Autodesk Inventor part; units mm, degrees
ref_plane "YZ Plane" through (0, 0, 0) normal (1, 0, 0) x (0, 1, 0)
ref_plane "XZ Plane" through (0, 0, 0) normal (0, 1, 0) x (-1, 0, 0)
ref_plane "XY Plane" through (0, 0, 0) normal (0, 0, 1) x (1, 0, 0)
sketch "Sketch1" plane through (0, 0, 0) normal (0, 1, 0) x (-1, 0, 0)
  line L0 (0, 0) -> (1219.2, 0)
  line L1 (1219.2, 0) -> (1219.2, -1219.2)
  line L2 (1219.2, -1219.2) -> (0, -1219.2)
  line L3 (0, -1219.2) -> (0, 0)
  dimension "d0" = 1219.2
  dimension "d1" = 1219.2
extrude "Extrusion1" add sketch "Sketch1" along normal blind 25.4
sketch "Sketch2" plane through (0, 25.4, 0) normal (0, 1, 0) x (1, 0, 0)
  line L0 (-790.7708, 108.1811) -> (-790.7708, 1049.4054)
  line L1 (-790.7708, 1049.4054) -> (-104.9708, 1049.4054)
  line L2 (-104.9708, 1049.4054) -> (-104.9708, 656.4029)
  line L3 (-104.9708, 656.4029) -> (-468.5932, 656.4029)
  line L4 (-468.5932, 656.4029) -> (-468.5932, 108.1811)
  line L5 (-468.5932, 108.1811) -> (-790.7708, 108.1811)
  point P0 (0, 0)
  dimension "d10" = 685.8
extrude "Extrusion2" add sketch "Sketch2" along normal blind 304.8
sketch "Sketch3" plane through (-104.9708, 25.4, -656.4029) normal (1, 0, 0) x (0, 0, -1)
  line L0 (-33.1569, 274.7838) -> (196.5012, 492.1801)
  line L1 (196.5012, 492.1801) -> (437.777, 274.7838)
  line L2 (437.777, 274.7838) -> (-33.1569, 274.7838)
  line L3 (0, 304.8) -> (393.0024, 304.8)
  point P0 (-656.4029, -25.4)
extrude "Extrusion3" add sketch "Sketch3" along normal blind 25.4
extrude "Extrusion4" add sketch "Sketch3" against normal blind 711.2
sketch "Sketch4" plane through (-790.7708, 25.4, -108.1811) normal (0, 0, 1) x (1, 0, 0)
  line L0 (-63.4257, 274.7838) -> (161.0888, 492.1801)
  line L1 (161.0888, 492.1801) -> (386.3126, 274.7838)
  line L2 (322.1776, 274.7838) -> (711.2, 274.7838)
  line L3 (-63.4257, 274.7838) -> (386.3126, 274.7838)
  line L4 (0, 304.8) -> (322.1776, 304.8)
  line L5 (711.2, 492.1801) -> (-25.4, 492.1801)
  point P0 (790.7708, -25.4)
extrude "Extrusion5" add sketch "Sketch4" against normal blind 744.22
extrude "Extrusion6" add sketch "Sketch4" along normal blind 25.4
sketch "Sketch5" plane through (0, 0, 0) normal (0, -1, 0) x (1, 0, 0)
  line L0 (-560.0074, -996.6268) -> (-666.9511, -996.6268)
  line L1 (-666.9511, -996.6268) -> (-666.9511, -948.1994)
  line L2 (-666.9511, -948.1994) -> (-560.0074, -948.1994)
  line L3 (-560.0074, -948.1994) -> (-560.0074, -996.6268)
  point P0 (0, 0)
extrude "Extrusion7" add sketch "Sketch5" against normal blind 508
equation "\"d1\" = d0"
properties part number "house_1" material "Wood (Oak)"
Design review of the part built by this model. Coordinates are the model's own, in mm. A direction names the side the tool comes from. Round coordinates to 2 decimals unless told otherwise and drop trailing zeros. Write each loop counter-clockwise with the first axis right and the second up, starting at its lowest first coordinate (ties: lowest second). Pieces come first, ordered by that corner, then holes. Notation, with made-up numbers: (50, -28.5) -> (61, -28.5) arc R35 cw to (61, 6.5) -> close; hole circle Ø10 at (24.25, -9.75). An arc over 180 degrees is marked (long way). One line per question, with ' | ' between items.
(1) Insertion check: P1, Ø8, axis at x = -728, y = 64, coming from the +Z side; P2, Ø14.5, axis at y = 425.5, z = -965, coming from the +X side; P3, Ø12, axis at y = 173, z = -135.5, coming from the -X side. Each pin has a flat end and moves straight along its axis. Give the tip position at first contact, or say it passes through.
Result sheet:
P1: z = -108.18 | P2: x = -79.57 | P3: x = -790.77
(2) Machinability: for faces 1 (the flat face through (-816.171, 386, -875)), 2 (the flat face through (-284, 161, -656.403)), 3 (the flat face through (-790.771, 161, -572)), 4 (the flat face through (-613, 447, -996.627)), which of the approach directions +Z, -Z, +X, -X, +Y, -Y give a long, thin tool a straight path to every point of the face, cutting with its end or side? Answer none if there is none.
Result sheet:
face 1: -Z, -X, +Y | face 2: +Z, +X | face 3: +Z, -Z, -X | face 4: -Z, +X, -X, +Y
(3) Take a section at A-A, the plane x = -263.5. State the section outline as (y, z) points.
Result sheet:
outline: (0, -1219.2) -> (25.4, -1219.2) -> (25.4, -1049.41) -> (300.18, -1049.41) -> (300.18, -1094.18) -> (517.58, -852.9) -> (300.18, -623.25) -> (300.18, -656.4) -> (25.4, -656.4) -> (25.4, 0) -> (0, 0) -> close
(4) Take a section at B-B, the plane z = -317. State the section outline as (x, y) points, and give its area (3 significant figures).
Result sheet:
outline: (-1219.2, 0) -> (0, 0) -> (0, 25.4) -> (-468.59, 25.4) -> (-468.59, 300.18) -> (-404.46, 300.18) -> (-629.68, 517.58) -> (-854.2, 300.18) -> (-790.77, 300.18) -> (-790.77, 25.4) -> (-1219.2, 25.4) -> close | area: 168,000 mm2
(5) Draft analysis for pull direction Y (two halves, no side actions). For faces 5 (the flat face through (-618, 0, -601)), 6 (the flat face through (-468.593, 161, -386)), 7 (the flat face through (-666.951, 461, -973)), state which applies: released by +Y, released by -Y, zero draft, split by the parting line, or undercut.
Result sheet:
face 5: released by -Y | face 6: undercut | face 7: zero draft
(6) Take a section at D-D, the plane z = -1142. State the section outline as (x, y) points.
Result sheet:
outline: (-1219.2, 0) -> (0, 0) -> (0, 25.4) -> (-1219.2, 25.4) -> close
(7) Take a section at C-C, the plane y = 91. State the section outline as (x, z) points.
Result sheet:
outline: (-790.77, -1049.41) -> (-104.97, -1049.41) -> (-104.97, -656.4) -> (-468.59, -656.4) -> (-468.59, -108.18) -> (-790.77, -108.18) -> close
(8) Wall thickness on line 1 (Z direction, x = -403, y = 65.5); line 2 (X direction, y = 248, z = -960.5); line 3 (Y direction, x = -355, z = -53): over which ranges is each line inside the solid? List them lowest first. Write a range as [from, to].
Result sheet:
line 1: [-1049.41, -656.4] | line 2: [-790.77, -104.97] | line 3: [0, 25.4]
